Here's the drawing with two shaded views (mm, measured from the low corner). I have some questions. A direction names the side the tool comes from. Coordinates: 2 decimals unless noted, no trailing zeros. Order: outer loops, then holes, each group sorted by start corner. A loop starts at its lowest first (then second) coordinate and runs counter-clockwise, first axis right, second up. Notation, with made-up numbers: (85.5, 45.25) -> (117.5, 45.25) arc R17 ccw to (117.5, 52.25) -> close; hole circle Ø4 at (86, 74). An arc over 180 degrees is marked (long way). Answer in a Markdown table with one row per item. Add a question column.
1. Imagine slicing it at B-B on x = 7.5. Write out the boundary of the cut face in (y, z), plus the area to 3 significant figures.
2. Will these pins go through, and if not, where does the flat tip stop? pin 1 (10 mm diameter, centred on y = 11.5, z = 34.5, fed in from -X); pin 2 (6 mm diameter, centred on y = 13.5, z = 24, fed in from +X); pin 3 (10 mm diameter, centred on x = 28.5, z = 25.5, fed in from -Y).
3. If I drill on line 1 along Y through (x, z) = (52.5, 7); line 2 along X through (y, z) = (16, 31); line 3 along X through (y, z) = (15.5, 45.5), over which ranges is the centre line in solid material (lowest first)? Write a range as [from, to].
4. Imagine slicing it at A-A on z = 31. Write out the boundary of the cut face in (x, y), plus the area to 3 significant figures.
5. We'd pull the mould along X, two halves only. Please class the marked faces 1, 2, 3 and 4: pulls with the +X half, pulls with the -X half, needs draft (parallel to the pull), parting line crosses it, or undercut.
6. On a 3-axis mill with a long thin cutter (end or side, diameter ignored), from which of +Z, -Z, +X, -X, +Y, -Y can I reach the whole of each face in a straight line? I mean the marked faces 5, 6 and 7. Say none if no direction works.
7. Imagine slicing it at D-D on x = 38. Write out the boundary of the cut face in (y, z).
8. Imagine slicing it at C-C on y = 13.75. Write out the boundary of the cut face in (x, z).
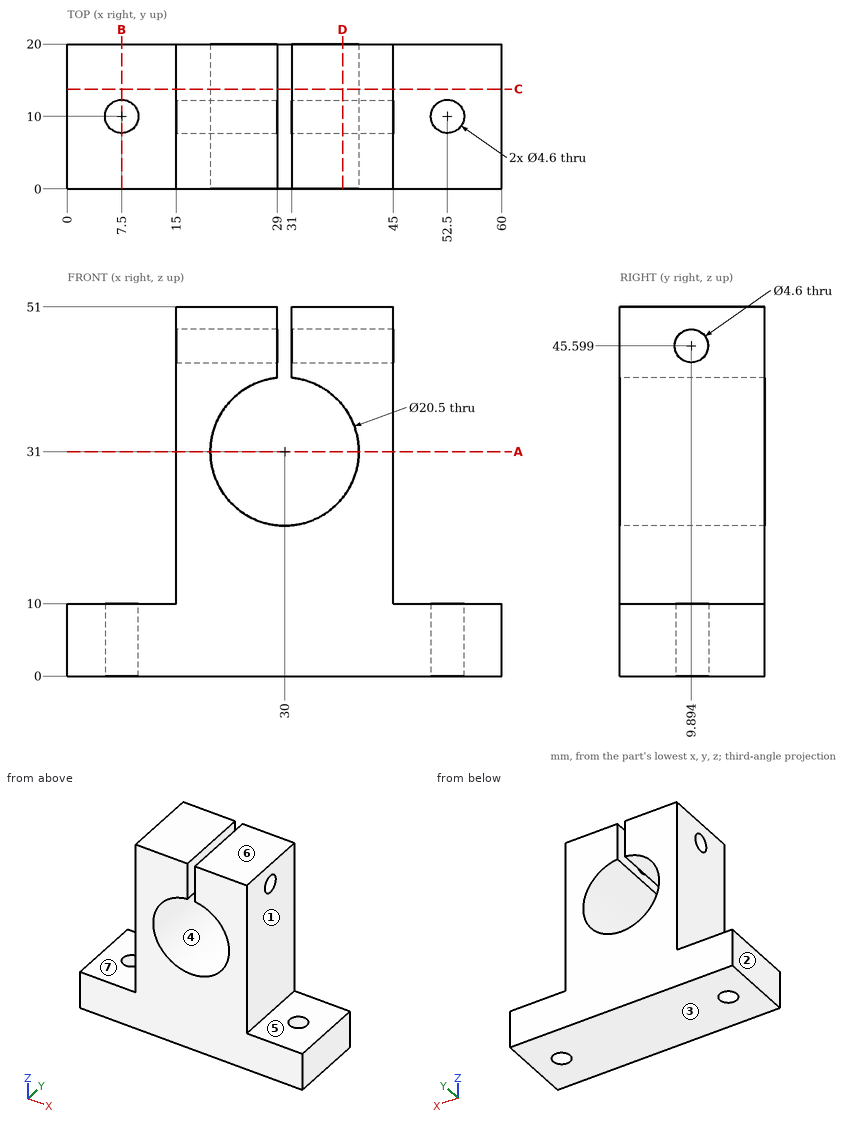
Answers follow:
| question | item | result |
|---|---|---|
| 1 | outline | (0, 0) -> (7.7, 0) -> (7.7, 10) -> (0, 10) -> close; (12.3, 0) -> (20, 0) -> (20, 10) -> (12.3, 10) -> close |
| 1 | area | 154 mm² |
| 2 | pin 1 | stops at x = 15 |
| 2 | pin 2 | stops at x = 45 |
| 2 | pin 3 | stops at y = 0 |
| 3 | line 1 | y = [0, 7.7], [12.3, 20] |
| 3 | line 2 | x = [15, 19.75], [40.25, 45] |
| 3 | line 3 | x = [15, 29], [31, 45] |
| 4 | outline | (15, 0) -> (19.75, 0) -> (19.75, 20) -> (15, 20) -> close; (40.25, 0) -> (45, 0) -> (45, 20) -> (40.25, 20) -> close |
| 4 | area | 190 mm² |
| 5 | face 1 | pulls with the +X half |
| 5 | face 2 | pulls with the -X half |
| 5 | face 3 | needs draft |
| 5 | face 4 | undercut |
| 6 | face 5 | +Z, +X, +Y, -Y |
| 6 | face 6 | +Z, +X, -X, +Y, -Y |
| 6 | face 7 | +Z, -X, +Y, -Y |
| 7 | outline | (0, 0) -> (20, 0) -> (20, 24.59) -> (0, 24.59) -> close; (0, 37.41) -> (20, 37.41) -> (20, 51) -> (0, 51) -> close; hole circle Ø4.6 at (9.89, 45.6) |
| 8 | outline | (0, 0) -> (60, 0) -> (60, 10) -> (45, 10) -> (45, 51) -> (31, 51) -> (31, 41.2) arc R10.25 cw (long way) to (29, 41.2) -> (29, 51) -> (15, 51) -> (15, 10) -> (0, 10) -> close |
